Could you check a few things on this model? Use its own coordinates, in mm. A direction names the side the tool comes from. Coordinates: 2 decimals unless noted, no trailing zeros. Write each loop counter-clockwise with the first axis right and the second up, starting at its lowest first coordinate (ties: lowest second). Pieces come first, ordered by that corner, then holes. Notation, with made-up numbers: (-12.75, 24) - (13.25, 24) arc R10 cw to (13.25, 35) - close; hole circle Ø7 at (-32.5, 79). An arc over 180 degrees is marked (long way). Answer as a JSON object with one key per item and string values. Group by question number.
1) If we section it at D-D (y = 0): Write out the boundary of the cut face in (x, z), plus the area to 4 significant figures.
2) If we section it at C-C (x = -16): Write out the boundary of the cut face in (y, z), plus the area to 3 significant figures.
3) We'd pull the mould along Y, two halves only. Please class faces 1 (the conical face through (-34.5, 0.2, 9.8)), 2 (the flat face through (-3, -31, 3.263)), 3 (the flat face through (-17, -25.7, 3)): released by +Y, released by -Y, zero draft, split by the parting line, or undercut.
4) If we section it at B-B (z = 4.25): Write out the boundary of the cut face in (x, y), plus the area to 3 significant figures.
5) If we section it at A-A (z = 0): Write out the boundary of the cut face in (x, y) (3 decimals).
6) Will these pins go through, and if not, where does the flat tip stop? pin 1 Ø6 at (x, z) = (-15, 5) entering from +Y; pin 2 Ø10 at (y, z) = (1.5, -7) entering from +X; pin 3 Ø10 at (y, z) = (31.3, 0) entering from -X; pin 4 Ø5 at (y, z) = (-31.3, 0) entering from +X.
7) Please list where these lines run through material, in increasing order: line 1 along Z through (x, y) = (-4.35, -31.3) (3 decimals); line 2 along Y through (x, z) = (-4.25, 0) (3 decimals); line 3 along Y through (x, z) = (-3.65, 0) (3 decimals).
8) On a 3-axis mill with a long thin cutter (end or side, diameter ignored), from which of +Z, -Z, +X, -X, +Y, -Y can I reach the whole of each face in a straight line? I mean faces 4 (the flat face through (-14.596, 28.089, -4.612)), 5 (the flat face through (-14.327, -28.461, -4.827)), 6 (the flat face through (0, -26, 0)), 7 (the flat face through (-3, 31, 3.263)). Say none if no direction works.
```python
from build123d import *

# Parameters (mm, degrees)
PAD007_DEPTH    = 10
SKETCH023_R     = 3.175
POCKET013_DEPTH = 208.8404998244
POCKET014_DEPTH = 208.8405005395
POCKET015_DEPTH = 32
CHAMFER005_SIZE = 3
SKETCH026_W     = 11.6
SKETCH026_H     = 13.2331615075
POCKET016_DEPTH = 32
SKETCH027_W     = 6
SKETCH027_H     = 3.1836615393
POCKET017_DEPTH = 32
CHAMFER006_SIZE = 1


with BuildPart() as part:
    # Sketch022 → Pad007 (new body, symmetric)
    with BuildSketch(Plane.XY):
        with BuildLine():
            ThreePointArc((0, 19.3), (-19.3, 0), (0, -19.3))
            Line((0, -19.3), (0, -37.3))
            ThreePointArc((0, 37.3), (-37.3, 0), (0, -37.3))
            Line((0, 37.3), (0, 19.3))
        make_face()
    extrude(amount=PAD007_DEPTH, both=True)

    # Sketch023 (on Face3 of Pad007) → Pocket013 (cut, through all)
    with BuildSketch(Plane.YZ):
        with Locations((-31.3, 0)):
            Circle(SKETCH023_R)
    pocket013 = extrude(amount=-POCKET013_DEPTH, mode=Mode.SUBTRACT)

    # Mirrored013: Pocket013 across Sketch023 V_Axis
    add(pocket013.mirror(Plane(origin=(0, 0, 0), x_dir=(1, 0, 0), z_dir=(0, 1, 0))), mode=Mode.SUBTRACT)

    # Sketch024 (on Face7 of Mirrored013) → Pocket014 (cut, through all)
    with BuildSketch(Plane.YZ):
        Polygon((-32.3, 3.0134075396), (-30.3, 3.0134075396), (-30.55, 3.2634075396), (-32.05, 3.2634075396), align=None)
    pocket014 = extrude(amount=-POCKET014_DEPTH, mode=Mode.SUBTRACT)

    # Mirrored014: Pocket014 across Sketch024 V_Axis
    add(pocket014.mirror(Plane(origin=(0, 0, 0), x_dir=(1, 0, 0), z_dir=(0, 1, 0))), mode=Mode.SUBTRACT)

    # Sketch025 (on DatumPlane) → Pocket015 (cut)
    with BuildSketch(Plane(origin=(-38, 0, 0), x_dir=(0, -1, 0), z_dir=(-1, 0, 0))):
        Polygon((31.3, 6.4663230149), (25.7, 3.2331615075), (25.7, -3.2331615075), (31.3, -6.4663230149), (36.9, -3.2331615075), (36.9, 3.2331615075), align=None)
    pocket015 = extrude(amount=-POCKET015_DEPTH, mode=Mode.SUBTRACT)

    # Mirrored015: Pocket015 across Sketch025 V_Axis
    add(pocket015.mirror(Plane(origin=(-38, 0, 0), x_dir=(-1, 0, 0), z_dir=(0, -1, 0))), mode=Mode.SUBTRACT)

    # Chamfer005
    chamfer005_edges = [part.edges().sort_by_distance(p)[0] for p in [
        (-37.3, 0, 10),
    ]]
    chamfer(chamfer005_edges, length=CHAMFER005_SIZE)

    # Sketch026 (on DatumPlane) → Pocket016 (cut)
    with BuildSketch(Plane(origin=(-38, 0, 0), x_dir=(0, -1, 0), z_dir=(-1, 0, 0))):
        with Locations((31.5, 3.3834192463)):
            Rectangle(SKETCH026_W, SKETCH026_H)
    pocket016 = extrude(amount=-POCKET016_DEPTH, mode=Mode.SUBTRACT)

    # Mirrored016: Pocket016 across Sketch026 V_Axis
    add(pocket016.mirror(Plane(origin=(-38, 0, 0), x_dir=(-1, 0, 0), z_dir=(0, -1, 0))), mode=Mode.SUBTRACT)

    # Sketch027 (on DatumPlane) → Pocket017 (cut)
    with BuildSketch(Plane(origin=(-38, 0, 0), x_dir=(0, -1, 0), z_dir=(-1, 0, 0))):
        with Locations((34.3, -4.8744922453)):
            Rectangle(SKETCH027_W, SKETCH027_H)
    pocket017 = extrude(amount=-POCKET017_DEPTH, mode=Mode.SUBTRACT)

    # Mirrored017: Pocket017 across Sketch027 V_Axis
    add(pocket017.mirror(Plane(origin=(-38, 0, 0), x_dir=(-1, 0, 0), z_dir=(0, -1, 0))), mode=Mode.SUBTRACT)

    # Chamfer006
    chamfer006_edges = [part.edges().sort_by_distance(p)[0] for p in [
        (-14.357817, -25.7, 10),
        (-6, -29.735571, 10),
        (-6, -35.293157, 8.500461),
        (-6, -36.814264, 0.266838),
        (-27.033313, 25.7, 1.883419),
        (-24.890244, 25.7, 8.522713),
        (-14.357817, 25.7, 10),
        (-6, 29.735571, 10),
        (-6, 35.293157, 8.500461),
        (-6, 36.814264, 0.266838),
    ]]
    chamfer(chamfer006_edges, length=CHAMFER006_SIZE)


solid = part.part
```
Here are the results:
{
 "1": {"outline": "(-37.3, -10) - (-19.3, -10) - (-19.3, 10) - (-34.3, 10) - (-37.3, 7) - close", "area": "355.5 mm²"},
 "2": {"outline": "(-33.69, -10) - (-10.79, -10) - (-10.79, 10) - (-24.7, 10) - (-25.7, 9) - (-25.7, -3.23) - (-31.3, -6.47) - (-33.69, -6.47) - close; (10.79, -10) - (33.69, -10) - (33.69, -6.47) - (31.3, -6.47) - (25.7, -3.23) - (25.7, 9) - (24.7, 10) - (10.79, 10) - close", "area": "670 mm²"},
 "3": {"face 1": "split by the parting line", "face 2": "undercut", "face 3": "released by -Y"},
 "4": {"outline": "(-27.71, 24.97) arc R37.3 ccw to (-27.03, -25.7) - (-6, -25.7) - (-6, -35.81) - (-5.01, -36.96) arc R37.3 ccw to (0, -37.3) - (0, -19.3) arc R19.3 cw to (0, 19.3) - (0, 37.3) arc R37.3 ccw to (-5.01, 36.96) - (-6, 35.81) - (-6, 25.7) - (-26.03, 25.7) - close", "area": "1,300 mm²"},
 "5": {"outline": "(-27.713, 24.966) arc R37.3 ccw to (-27.033, -25.7) - (-6, -25.7) - (-6, -28.125) - (0, -28.125) - (0, -19.3) arc R19.3 cw to (0, 19.3) - (0, 28.125) - (-6, 28.125) - (-6, 25.7) - (-26.033, 25.7) - close; (-6, -35.814) - (-5.011, -36.962) arc R37.3 ccw to (0, -37.3) - (0, -34.475) - (-6, -34.475) - close; (-6, 34.475) - (0, 34.475) - (0, 37.3) arc R37.3 ccw to (-5.011, 36.962) - (-6, 35.814) - close"},
 "6": {"pin 1": "stops at y = 25.7", "pin 2": "stops at x = -18.17", "pin 3": "stops at x = -6", "pin 4": "passes through"},
 "7": {"line 1": "z = -10 to -3.175, 3.263 to 10", "line 2": "y = -37.057 to -34.475, -28.125 to -18.826, 18.826 to 28.125, 34.475 to 37.057", "line 3": "y = -37.121 to -34.475, -28.125 to -18.952, 18.952 to 28.125, 34.475 to 37.121"},
 "8": {"face 4": "+Z, -X, +Y", "face 5": "+Z, -X, -Y", "face 6": "+Z, -Z, +X, +Y, -Y", "face 7": "+X, -X"}
}
